Check sheet for the drawn part. Datum: minimum x, y, z corner. Units: mm. Coordinates: 2 decimals unless noted, no trailing zeros. Loops run counter-clockwise (first coordinate to the right, second up) from the corner with the lowest first, then second, coordinate; pieces in that order, holes last.
Q1. Sectioned sample at B-B (z = 2.1). Enter the section's corners in (x, y).
Q2. Sectioned sample at C-C (x = 163). Enter the section's corners in (y, z), then the cut area to 3 significant figures.
Q3. Material ranges on probe 1 along X at (y, z) = (28, 0.6); probe 2 along Y at (x, z) = (72.5, 2.3), recorded low to high.
Q4. Go/stop test with flat-tipped pins: P1, Ø1, axis at y = 1, z = 1, coming from the -X side; P2, Ø1, axis at x = 168.5, z = 1.5, coming from the -Y side; P3, Ø1, axis at y = 1.5, z = 2.5, coming from the +X side. Record where each tip stops, or that it passes through.
Q5. Sectioned sample at A-A (y = 33.5). Enter the section's corners in (x, z), then the cut area to 3 significant figures.
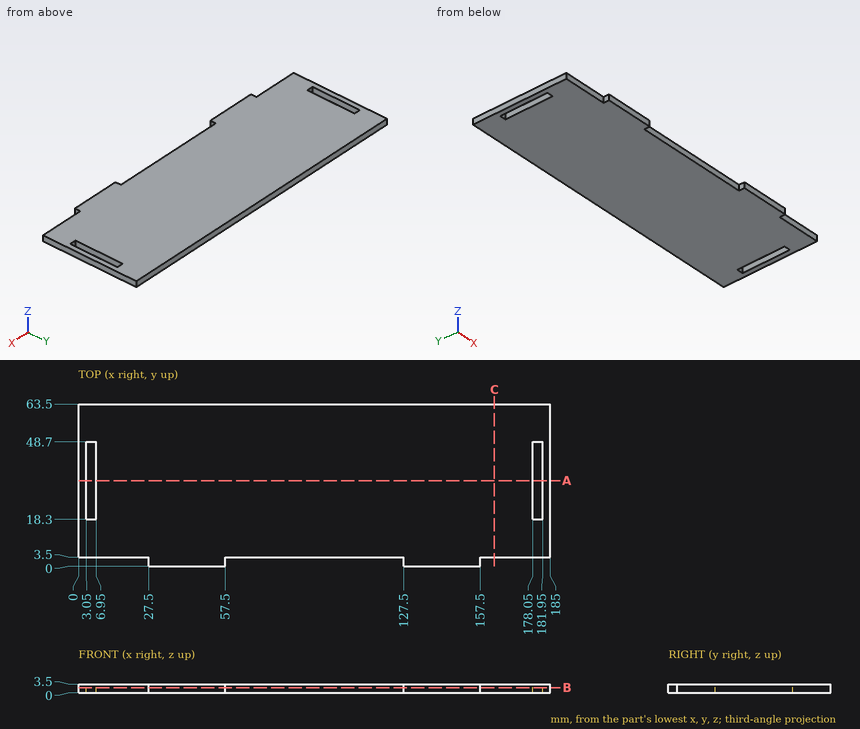
Geometry check:
1. outline: (0, 3.5) - (27.5, 3.5) - (27.5, 0) - (57.5, 0) - (57.5, 3.5) - (127.5, 3.5) - (127.5, 0) - (157.5, 0) - (157.5, 3.5) - (185, 3.5) - (185, 63.5) - (0, 63.5) - close; hole (3.05, 18.3) - (6.95, 18.3) - (6.95, 48.7) - (3.05, 48.7) - close; hole (178.05, 18.3) - (181.95, 18.3) - (181.95, 48.7) - (178.05, 48.7) - close
2. outline: (3.5, 0) - (63.5, 0) - (63.5, 3.5) - (3.5, 3.5) - close
2. area: 210 mm2
3. probe 1: x = 0 to 3.05, 6.95 to 178.05, 181.95 to 185
3. probe 2: y = 3.5 to 63.5
4. P1: stops at x = 27.5
4. P2: stops at y = 3.5
4. P3: stops at x = 157.5
5. outline: (0, 0) - (3.05, 0) - (3.05, 3.5) - (0, 3.5) - close; (6.95, 0) - (178.05, 0) - (178.05, 3.5) - (6.95, 3.5) - close; (181.95, 0) - (185, 0) - (185, 3.5) - (181.95, 3.5) - close
5. area: 620 mm2
